```python
from build123d import *

# Parameters (mm, degrees)
BOSS_EXTRUDE1_DEPTH      = 50
SKETCH3_R                = 50
CUT_EXTRUDE1_DEPTH       = 50
BOSS_EXTRUDE2_START      = 25
BOSS_EXTRUDE2_DEPTH      = 5
FILLET1_R                = 10
SKETCH6_R                = 100
CUT_EXTRUDE2_DEPTH       = 12.5
BOSS_EXTRUDE3_START      = -26
SKETCH7_R                = 6
BOSS_EXTRUDE3_DEPTH      = 51
CIRPATTERN1_COUNT        = 3
CIRPATTERN1_START        = 25
CIRPATTERN1_COPY_1_DEPTH = 5
CIRPATTERN1_COPY_2_DEPTH = 5


with BuildPart() as part:
    # Sketch1 → Boss-Extrude1 (new body)
    with BuildSketch(Plane(origin=(0, 0, 0), x_dir=(1, 0, 0), z_dir=(0, 1, 0))):
        with BuildLine():
            Line((0, 150), (-30, 150))
            Line((-30, 150), (-30, 121.346610995))
            ThreePointArc((-30, 121.346610995), (-108.253175473, 62.5), (-120.089247785, -34.692543384))
            Line((-120.089247785, -34.692543384), (-144.903810568, -49.019237886))
            Line((-144.903810568, -49.019237886), (-129.903810568, -75))
            Line((-129.903810568, -75), (-114.903810568, -100.980762114))
            Line((-114.903810568, -100.980762114), (-90.089247785, -86.654067611))
            ThreePointArc((-90.089247785, -86.654067611), (0, -125), (90.089247785, -86.654067611))
            Line((90.089247785, -86.654067611), (114.903810568, -100.980762114))
            Line((114.903810568, -100.980762114), (129.903810568, -75))
            Line((129.903810568, -75), (144.903810568, -49.019237886))
            Line((144.903810568, -49.019237886), (120.089247785, -34.692543384))
            ThreePointArc((120.089247785, -34.692543384), (108.253175473, 62.5), (30, 121.346610995))
            Line((30, 121.346610995), (30, 150))
            Line((30, 150), (0, 150))
        make_face()
    extrude(amount=BOSS_EXTRUDE1_DEPTH)

    # Sketch3 → Cut-Extrude1 (cut)
    with BuildSketch(Plane(origin=(0, 50, 0), x_dir=(1, 0, 0), z_dir=(0, 1, 0))):
        Circle(SKETCH3_R)
    extrude(amount=-CUT_EXTRUDE1_DEPTH, mode=Mode.SUBTRACT)

    # Sketch4 → Boss-Extrude2 (add)
    with BuildSketch(Plane(origin=(0, 0, 0), x_dir=(0, 0, -1), z_dir=(1, 0, 0)).offset(BOSS_EXTRUDE2_START)):
        with BuildLine():
            Line((150, 37.5), (220, 37.5))
            ThreePointArc((220, 37.5), (232.5, 25), (220, 12.5))
            Line((220, 12.5), (150, 12.5))
            ThreePointArc((150, 12.5), (137.5, 25), (150, 37.5))
        make_face()
    boss_extrude2 = extrude(amount=BOSS_EXTRUDE2_DEPTH)

    # Mirror1: Boss-Extrude2 across plane
    add(boss_extrude2.mirror(Plane(origin=(0, 0, 0), x_dir=(0, 0, 1), z_dir=(1, 0, 0))))

    # Fillet1
    fillet1_edges = [part.edges().sort_by_distance(p)[0] for p in [
        (-129.903810568, 50, 75),
        (0, 0, -150),
        (129.903810568, 0, 75),
        (-129.903810568, 0, 75),
        (129.903810568, 50, 75),
        (0, 50, -150),
    ]]
    fillet(fillet1_edges, radius=FILLET1_R)

    # Sketch6 → Cut-Extrude2 (cut)
    with BuildSketch(Plane(origin=(0, 50, 0), x_dir=(1, 0, 0), z_dir=(0, 1, 0))):
        Circle(SKETCH6_R)
    extrude(amount=-CUT_EXTRUDE2_DEPTH, mode=Mode.SUBTRACT)

    # Sketch7 → Boss-Extrude3 (add)
    with BuildSketch(Plane(origin=(0, 0, 0), x_dir=(0, 0, -1), z_dir=(1, 0, 0)).offset(BOSS_EXTRUDE3_START)):
        with Locations((220, 25)):
            Circle(SKETCH7_R)
    boss_extrude3 = extrude(amount=BOSS_EXTRUDE3_DEPTH)

    # CirPattern1: Boss-Extrude3, Boss-Extrude2 ×3 about axis
    cirpattern1_axis = Axis((0, 0, 0), (0, 1, 0))
    for i in range(1, CIRPATTERN1_COUNT):
        add(boss_extrude3.rotate(cirpattern1_axis, i * 360 / CIRPATTERN1_COUNT))
        add(boss_extrude2.rotate(cirpattern1_axis, i * 360 / CIRPATTERN1_COUNT))

    # CirPattern1 copy 1 sketch → CirPattern1 copy 1 (add)
    with BuildSketch(Plane(origin=(0, 0, 0), x_dir=(-0.866025404, 0, 0.5), z_dir=(0.5, 0, 0.866025404)).offset(CIRPATTERN1_START)):
        with BuildLine():
            Line((150, -37.5), (220, -37.5))
            ThreePointArc((220, -37.5), (232.5, -25), (220, -12.5))
            Line((220, -12.5), (150, -12.5))
            ThreePointArc((150, -12.5), (137.5, -25), (150, -37.5))
        make_face()
    extrude(amount=CIRPATTERN1_COPY_1_DEPTH)

    # CirPattern1 copy 2 sketch → CirPattern1 copy 2 (add)
    with BuildSketch(Plane(origin=(0, 0, 0), x_dir=(0.866025404, 0, 0.5), z_dir=(0.5, 0, -0.866025404)).offset(CIRPATTERN1_START)):
        with BuildLine():
            Line((150, -37.5), (220, -37.5))
            ThreePointArc((220, -37.5), (232.5, -25), (220, -12.5))
            Line((220, -12.5), (150, -12.5))
            ThreePointArc((150, -12.5), (137.5, -25), (150, -37.5))
        make_face()
    extrude(amount=CIRPATTERN1_COPY_2_DEPTH)


solid = part.part
```
For this review, take the finished solid that the model builds, in its own axes (mm). A direction names the side the tool comes from. Round coordinates to 2 decimals unless told otherwise and drop trailing zeros. Write each loop counter-clockwise with the first axis right and the second up, starting at its lowest first coordinate (ties: lowest second). Pieces come first, ordered by that corner, then holes. Notation, with made-up numbers: (60, 35) - (95, 35) arc R15 ccw to (95, 39) - close; hole circle Ø10 at (-39, -10). An arc over 180 degrees is marked (long way). Answer as CSV lines item,"result". Start each with the question number.
(1) Add section C-C, the plane x = 77.5. State the section outline as (y, z) points.
(2) For pin 1 (1 mm diameter, centred on y = 23, z = 74.5, fed in from +X); pin 2 (5 mm diameter, centred on x = -56, y = 15.5, fed in from +Z); pin 3 (4 mm diameter, centred on y = 16.5, z = -157.5, fed in from +X), all flat-tipped, find the tip position at first contact; note any pin that passes through.
(3) Add section B-B, the plane x = -5.5. State the section outline as (y, z) points, plus the area to 3 significant figures.
(4) Mouldability with a two-part tool opening along Z and no side actions: class faces 4 (the cylindrical face through (95.38, 43.84, -30.04)), 5 (the cylindrical face through (215.081, 25.275, 92.463)), 6 (the flat face through (-146, 37.5, 116)) as +Z half, -Z half, draft (parallel to the pull), parting line (faces both ways), or undercut.
(5) Add section D-D, the plane z = 67. State how many separate pieces and enclosed holes the cut face has, plus the area to 3 significant figures.
(6) Machinability: for faces 1 (the cylindrical face through (187.62, 25.27, 140.03)), 2 (the flat face through (-30, 25, -165)), 3 (the cylindrical face through (-0.35, 26.802, -225.723)), which of the approach directions +Z, -Z, +X, -X, +Y, -Y give a long, thin tool a straight path to every point of the face, cutting with its end or side? Answer none if there is none.
(7) Add section A-A, the plane z = 16.5. State the section outline as (x, y) points, plus the area to 3 significant figures.
(8) For line 1 (X direction, y = 45.75, z = 0); line 2 (X direction, y = 14.5, z = 0); line 3 (X direction, y = 30, z = 113), list the stretches that pass through material, from the lowest coordinate up.
From the geometry:
1,outline,"(0, -98.08) - (50, -98.08) - (50, -63.2) - (37.5, -63.2) - (37.5, 63.2) - (50, 63.2) - (50, 98.08) - (0, 98.08) - close"
2,pin 1,"stops at x = 189.9"
2,pin 2,"stops at z = 112.97"
2,pin 3,"stops at x = 30"
3,outline,"(0, -140) arc R10 ccw to (10, -150) - (40, -150) arc R10 ccw to (50, -140) - (50, -99.85) - (37.5, -99.85) - (37.5, -49.7) - (0, -49.7) - close; (0, 49.7) - (37.5, 49.7) - (37.5, 99.85) - (50, 99.85) - (50, 124.88) - (0, 124.88) - close; circle Ø12 at (25, -220)"
3,area,"7,590 mm²"
4,face 4,"undercut"
4,face 5,"+Z half"
4,face 6,"draft"
5,separate pieces,"3"
5,enclosed holes,"0"
5,area,"12,000 mm²"
6,face 1,"+Z, +X"
6,face 2,"-Z, -X, +Y, -Y"
6,face 3,"none"
7,outline,"(-123.91, 0) - (-47.2, 0) - (-47.2, 37.5) - (-98.63, 37.5) - (-98.63, 50) - (-123.91, 50) - close; (47.2, 0) - (123.91, 0) - (123.91, 50) - (98.63, 50) - (98.63, 37.5) - (47.2, 37.5) - close"
7,area,"6,380 mm²"
8,line 1,"x = -125 to -100, 100 to 125"
8,line 2,"x = -125 to -50, 50 to 125"
8,line 3,"x = -192.62 to -184.96, -145.72 to -135.72, -53.44 to 53.44, 135.72 to 145.72, 184.96 to 192.62"
